For this review, take the finished solid that the model builds, in its own axes (mm). A direction names the side the tool comes from. Round coordinates to 2 decimals unless told otherwise and drop trailing zeros. One line per question, with ' | ' between items.
```python
from build123d import *

# Parameters (mm, degrees)
SKETCH1_R           = 2
BOSS_EXTRUDE1_DEPTH = 243


with BuildPart() as part:
    # Sketch1 → Boss-Extrude1 (new body)
    with BuildSketch(Plane.XY):
        Polygon((6.4, 7.156263811), (4.243736189, 5), (5, 5), (5, 4.243736189), (7.156263811, 6.4), (9.056263811, 6.4), (9.056263811, 5), (10, 5), (10, 10), (5, 10), (5, 9.056263811), (6.4, 9.056263811), align=None)
        Polygon((-5, 0.245745613), (-5, 5), (-0.245745613, 5), (0, 4.827927069), (0.245745613, 5), (5, 5), (5, 0.245745613), (4.827927069, 0), (5, -0.245745613), (5, -5), (0.245745613, -5), (0, -4.827927069), (-0.245745613, -5), (-5, -5), (-5, -0.245745613), (-4.827927069, 0), align=None)
        Circle(SKETCH1_R, mode=Mode.SUBTRACT)
        Polygon((-10, 10), (-10, 5), (-9.056263811, 5), (-9.056263811, 6.4), (-7.156263811, 6.4), (-5, 4.243736189), (-5, 5), (-4.243736189, 5), (-6.4, 7.156263811), (-6.4, 9.056263811), (-5, 9.056263811), (-5, 10), align=None)
        Polygon((-5, -5), (-5, -4.243736189), (-7.156263811, -6.4), (-9.056263811, -6.4), (-9.056263811, -5), (-10, -5), (-10, -10), (-5, -10), (-5, -9.056263811), (-6.4, -9.056263811), (-6.4, -7.156263811), (-4.243736189, -5), align=None)
        Polygon((5, -5), (4.243736189, -5), (6.4, -7.156263811), (6.4, -9.056263811), (5, -9.056263811), (5, -10), (10, -10), (10, -5), (9.056263811, -5), (9.056263811, -6.4), (7.156263811, -6.4), (5, -4.243736189), align=None)
    extrude(amount=BOSS_EXTRUDE1_DEPTH)


solid = part.part
```
(1) Mouldability with a two-part tool opening along X and no side actions: class faces 1 (the flat face through (-10, 8, 120)), 2 (the flat face through (-2, -5, 120)), 3 (the flat face through (5, -2, 120)) as released by +X, released by -X, zero draft, split by the parting line, or undercut.
Output values:
face 1: released by -X | face 2: undercut | face 3: released by +X
(2) For faces 4 (the flat face through (-2, 5, 120)), 5 (the flat face through (2, -5, 120)), 6 (the flat face through (5, 2, 120)), 7 (the flat face through (-5, 2, 120)), list the 3-axis set-ups (+Z, -Z, +X, -X, +Y, -Y) from which the entire face can be reached by the end or side of a thin tool; tool diameter is ignored.
Output values:
face 4: +Z, -Z, +Y | face 5: +Z, -Z, -Y | face 6: +Z, -Z, +X | face 7: +Z, -Z, -X
(3) Insertion check: pin 1 (1.2 mm diameter, centred on x = 2.5, z = 169, fed in from +Y); pin 2 (1.5 mm diameter, centred on y = -1.5, z = 49.5, fed in from -X); pin 3 (1.5 mm diameter, centred on x = -1, z = 143.5, fed in from -Y). Each pin has a flat end and moves straight along its axis. Give the tip position at first contact, or say it passes through.
Output values:
pin 1: y = 5 | pin 2: x = -5 | pin 3: y = -5
(4) For probe 1 along X at (y, z) = (-9, 138.5); probe 2 along Y at (x, z) = (0, 189), list the stretches that pass through material, from the lowest coordinate up. Write a range as [from, to].
Output values:
probe 1: [-10, -6.4], [6.4, 10] | probe 2: [-4.83, -2], [2, 4.83]
